from build123d import *

# Parameters (mm, degrees)
F1_DEPTH = 12.7


with BuildPart() as f1:
    # F0 (on Front) → F1 (new body)
    with BuildSketch(Plane.XZ):
        with BuildLine():
            Line((373.228805, 321.540359), (0, 321.540359))
            Line((0, 321.540359), (-373.228805, 321.540359))
            ThreePointArc((-373.228805, 321.540359), (-446.77487, 302.619706), (-502.059262, 250.555796))
            Line((-502.059262, 250.555796), (-616.504222, 69.459962))
            ThreePointArc((-616.504222, 69.459962), (-625.738174, 9.20133), (-587.833517, -38.543886))
            Line((-587.833517, -38.543886), (-151.597384, -270.251901))
            ThreePointArc((-151.597384, -270.251901), (-116.945137, -283.540709), (-80.108337, -288.059641))
            Line((-80.108337, -288.059641), (80.108337, -288.059641))
            ThreePointArc((80.108337, -288.059641), (116.945137, -283.540709), (151.597384, -270.251901))
            Line((151.597384, -270.251901), (587.833517, -38.543886))
            ThreePointArc((587.833517, -38.543886), (625.738174, 9.20133), (616.504222, 69.459962))
            Line((616.504222, 69.459962), (502.059262, 250.555796))
            ThreePointArc((502.059262, 250.555796), (446.77487, 302.619706), (373.228805, 321.540359))
        make_face()
    extrude(amount=F1_DEPTH)


solid = f1.part
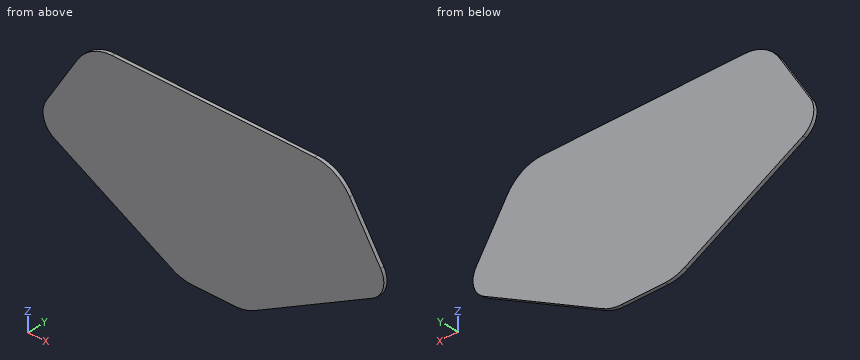
The listing builds one solid part. Answer for the finished solid, in the listing's coordinates (mm). Give positions to 0.01 mm unless a question says otherwise; leave off trailing zeros. Loops run counter-clockwise (first coordinate to the right, second up) from the corner with the lowest first, then second, coordinate; pieces in that order, holes last.
Item 1: Each of these flat-tipped pins is pushed along its axis until it touches: pin 1 Ø4 at (x, y) = (-426.5, -9.5) entering from +Z; pin 2 Ø4 at (x, z) = (304.5, 213.5) entering from +Y; pin 3 Ø5 at (y, z) = (-1.5, 38) entering from +X. Where does it stop, or does it pass through?
Derived:
pin 1: stops at z = 312.66
pin 2: stops at y = 0
pin 3: stops at x = 627.99
Item 2: A cutting plane is placed at C-C (x = 352.5). Give the vertices of the cut face in (y, z), then the cut area to 3 significant figures.
Derived:
outline: (-12.7, -163.54) - (0, -163.54) - (0, 321.54) - (-12.7, 321.54) - close
area: 6,160 mm2
Item 3: A cutting plane is placed at B-B (z = -166). Give the vertices of the cut face in (x, y).
Derived:
outline: (-347.87, -12.7) - (347.87, -12.7) - (347.87, 0) - (-347.87, 0) - close
Item 4: A cutting plane is placed at A-A (y = -4). Give the vertices of the cut face in (x, z), then the cut area to 3 significant figures.
Derived:
outline: (-616.5, 69.46) arc R76.2 ccw to (-587.83, -38.54) - (-151.6, -270.25) arc R152.4 ccw to (-80.11, -288.06) - (80.11, -288.06) arc R152.4 ccw to (151.6, -270.25) - (587.83, -38.54) arc R76.2 ccw to (616.5, 69.46) - (502.06, 250.56) arc R152.4 ccw to (373.23, 321.54) - (-373.23, 321.54) arc R152.4 ccw to (-502.06, 250.56) - close
area: 578,000 mm2
Item 5: Find the intervals of material crossed by line 1 along X through (y, z) = (-6.5, 25.5); line 2 along X through (y, z) = (-9.5, -8); line 3 along Z through (x, y) = (-286.5, -3.75), in increasing order.
Derived:
line 1: x = -628.22 to 628.22
line 2: x = -618.84 to 618.84
line 3: z = -198.6 to 321.54
